Read the model definition and answer for the solid it produces. Units are mm, in the model's axes. Face numbers are marked on the shaded views. Round coordinates to 2 decimals unless told otherwise and drop trailing zeros. Order: outer loops, then holes, each group sorted by start corner. A loop starts at its lowest first (then second) coordinate and runs counter-clockwise, first axis right, second up. Notation, with made-up numbers: (0, 5.5) -> (22, 5.5) arc R17 ccw to (22, 30.5) -> close; hole circle Ø9 at (41, 50). An arc over 180 degrees is marked (long way). One line per item, written item: value. Start each with the question number.
1. Section B-B (z = 1.55) is taken. Give the vertices of the cut face in (x, y).
2. Section C-C (y = 150) is taken. Give the vertices of the cut face in (x, z), then the cut area to 3 significant figures.
3. Section A-A (x = 216) is taken. Give the vertices of the cut face in (y, z).
4. Consider line 1 (X direction, y = 26, z = 1.75); line 2 (Y direction, x = 16, z = 1.55); line 3 (Y direction, x = 216, z = 2.2). Determine where each line is inside the solid, lowest interval first.
5. The mould has two halves that part along Z. Classify the marked faces 1 and 2: released by +Z, released by -Z, zero draft, split by the parting line, or undercut.
Autodesk Inventor part; units mm, degrees
ref_plane "YZ Plane" through (0, 0, 0) normal (1, 0, 0) x (0, 1, 0)
ref_plane "XZ Plane" through (0, 0, 0) normal (0, 1, 0) x (-1, 0, 0)
ref_plane "XY Plane" through (0, 0, 0) normal (0, 0, 1) x (1, 0, 0)
sketch "Sketch1" plane through (0, 0, 0) normal (0, 0, 1) x (1, 0, 0)
  line L0 (0, 0) -> (432, 0)
  line L1 (432, 0) -> (432, 642)
  line L2 (432, 642) -> (0, 642)
  line L3 (0, 642) -> (0, 0)
  line L4 (16, 626) -> (16, 26) construction
  line L5 (416, 626) -> (416, 26) construction
  line L6 (16, 626) -> (416, 626) construction
  line L7 (16, 26) -> (416, 26) construction
  circle A0 centre (216, 150) radius 50
  dimension "d0" = 432
  dimension "d1" = 642
  dimension "d2" = 600
  dimension "d3" = 400
  dimension "d4" = 16
  dimension "d5" = 16
  dimension "d6" = 100
  dimension "d7" = 150
  dimension "d8" = 216
extrude "Extrusion1" add sketch "Sketch1" along normal blind 3
hole "Hole1" at (16, 626, 0) at (416, 626, 0) at (416, 26, 0) at (16, 26, 0) direction (0, 0, 1) diameter 6.4 end through all
properties part number "top-ventilation-hole-100mm"
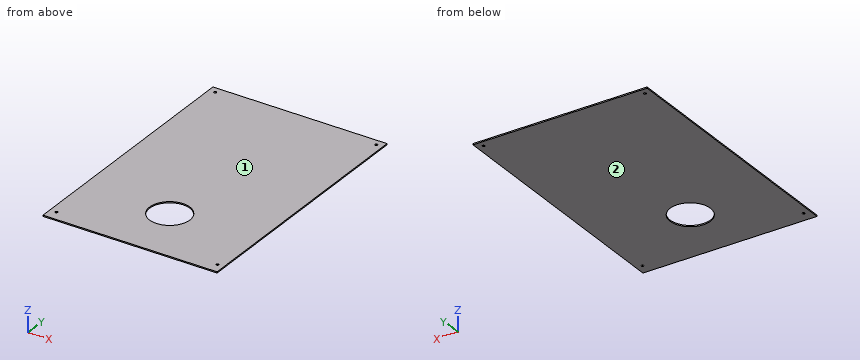
Answer:
1. outline: (0, 0) -> (432, 0) -> (432, 642) -> (0, 642) -> close; hole circle Ø6.4 at (16, 26); hole circle Ø6.4 at (16, 626); hole circle Ø100 at (216, 150); hole circle Ø6.4 at (416, 26); hole circle Ø6.4 at (416, 626)
2. outline: (0, 0) -> (166, 0) -> (166, 3) -> (0, 3) -> close; (266, 0) -> (432, 0) -> (432, 3) -> (266, 3) -> close
2. area: 996 mm^2
3. outline: (0, 0) -> (100, 0) -> (100, 3) -> (0, 3) -> close; (200, 0) -> (642, 0) -> (642, 3) -> (200, 3) -> close
4. line 1: 0 to 12.8, 19.2 to 412.8, 419.2 to 432
4. line 2: 0 to 22.8, 29.2 to 622.8, 629.2 to 642
4. line 3: 0 to 100, 200 to 642
5. face 1: released by +Z
5. face 2: released by -Z
